from build123d import *

# Parameters (mm, degrees)
CYLINDER016_R          = 3
CYLINDER016_DEPTH      = 20
CYLINDER016_ROLL_ANGLE = 90
CYLINDER015_R          = 3
CYLINDER015_DEPTH      = 20
CYLINDER015_ROLL_ANGLE = 90
BOX016_W               = 40
BOX016_H               = 40
BOX016_DEPTH           = 25
BOX016_ROLL_ANGLE      = 90


with BuildPart() as cylinder016:
    # Cylinder016 → Cylinder016 (new body)
    with BuildSketch(Plane.XY):
        Circle(CYLINDER016_R)
    extrude(amount=CYLINDER016_DEPTH)


with BuildPart() as cylinder016_1:
    # Cylinder016 roll: moved
    add(cylinder016.part.rotate(Axis((0, 0, 0), (1, 0, 0)), CYLINDER016_ROLL_ANGLE))


with BuildPart() as cylinder016_2:
    # Cylinder016 placement: moved
    add(cylinder016_1.part.moved(Location((162, -7, 145))))


with BuildPart() as cylinder015:
    # Cylinder015 → Cylinder015 (new body)
    with BuildSketch(Plane.XY):
        Circle(CYLINDER015_R)
    extrude(amount=CYLINDER015_DEPTH)


with BuildPart() as cylinder015_1:
    # Cylinder015 roll: moved
    add(cylinder015.part.rotate(Axis((0, 0, 0), (1, 0, 0)), CYLINDER015_ROLL_ANGLE))


with BuildPart() as cylinder015_2:
    # Cylinder015 placement: moved
    add(cylinder015_1.part.moved(Location((178, -7, 145))))


with BuildPart() as cut009:
    # Box016 → Box016 (new body)
    with BuildSketch(Plane.XY):
        with Locations((20, 20)):
            Rectangle(BOX016_W, BOX016_H)
    extrude(amount=BOX016_DEPTH)


with BuildPart() as cut009_1:
    # Box016 roll: moved
    add(cut009.part.rotate(Axis((0, 0, 0), (1, 0, 0)), BOX016_ROLL_ANGLE))


with BuildPart() as cut009_2:
    # Box016 placement: moved
    add(cut009_1.part.moved(Location((150, 0, 125))))

    # Cut008: cut Cylinder015
    add(cylinder015_2.part, mode=Mode.SUBTRACT)

    # Cut009: cut Cylinder016
    add(cylinder016_2.part, mode=Mode.SUBTRACT)


with BuildPart() as cut009_3:
    # Cut009 placement: moved
    add(cut009_2.part.moved(Location((0, 20, 0))))


solid = cut009_3.part
Source: CAD feature listing. Evaluate the final solid. Frame: model axes, mm. A direction names the side the tool comes from. Give positions to 0.01 mm unless a question says otherwise; leave off trailing zeros. Order: outer loops, then holes, each group sorted by start corner. A loop starts at its lowest first (then second) coordinate and runs counter-clockwise, first axis right, second up. Notation, with made-up numbers: (-36.75, 35) -> (17.25, 35) arc R22 cw to (17.25, 54) -> close; hole circle Ø7 at (57.25, 67.5). An arc over 180 degrees is marked (long way). Use a Markdown table: item, result.
1) Reachability of faces 5 (the flat face through (150, 8, 145)), 6 (the flat face through (162, 13, 145)) from +Z, -Z, +X, -X, +Y, -Y: full face, straight path, thin tool, end or side. Return the list, or none.
Answer list:
| item | result |
|---|---|
| face 5 | +Z, -Z, -X, +Y, -Y |
| face 6 | -Y |
2) Section query A-A, the plane z = 145. Return the cut outline in (x, y).
Answer list:
| item | result |
|---|---|
| outline | (150, -5) -> (159, -5) -> (159, 13) -> (165, 13) -> (165, -5) -> (175, -5) -> (175, 13) -> (181, 13) -> (181, -5) -> (190, -5) -> (190, 20) -> (150, 20) -> close |
3) Section query B-B, the plane y = -1.5. Return the cut outline in (x, z), then the cut area to 3 significant figures.
Answer list:
| item | result |
|---|---|
| outline | (150, 125) -> (190, 125) -> (190, 165) -> (150, 165) -> close; hole circle Ø6 at (162, 145); hole circle Ø6 at (178, 145) |
| area | 1,540 mm² |
4) Section query D-D, the plane x = 176. Return the cut outline in (y, z), then the cut area to 4 significant figures.
Answer list:
| item | result |
|---|---|
| outline | (-5, 125) -> (20, 125) -> (20, 165) -> (-5, 165) -> (-5, 147.24) -> (13, 147.24) -> (13, 142.76) -> (-5, 142.76) -> close |
| area | 919.5 mm² |
5) Section query C-C, the plane x = 162. Return the cut outline in (y, z), then the cut area to 3 significant figures.
Answer list:
| item | result |
|---|---|
| outline | (-5, 125) -> (20, 125) -> (20, 165) -> (-5, 165) -> (-5, 148) -> (13, 148) -> (13, 142) -> (-5, 142) -> close |
| area | 892 mm² |
6) Contact query for flat-ended pins moving along their axis: P1, Ø3.5, axis at x = 162, z = 145, coming from the -Y side; P2, Ø7, axis at x = 178, z = 145, coming from the -Y side. Output: stop coordinate, or through.
Answer list:
| item | result |
|---|---|
| P1 | y = 13 |
| P2 | y = -5 |
7) Ray query, line 1 along X through (y, z) = (4.75, 145); line 2 along Z through (x, y) = (162, -1.5); line 3 along Z through (x, y) = (160, 7). Return the intervals inside material, ascending. Write a range as [from, to].
Answer list:
| item | result |
|---|---|
| line 1 | [150, 159], [165, 175], [181, 190] |
| line 2 | [125, 142], [148, 165] |
| line 3 | [125, 142.76], [147.24, 165] |
8) Mould query, pull axis Z, two halves, no side actions, for faces 1 (the flat face through (170, 8, 165)), 2 (the flat face through (170, 8, 125)), 3 (the flat face through (170, -5, 145)), 4 (the cylindrical face through (163.61, 4.13, 147.53)). Classes: +Z half, -Z half, draft (parallel to the pull), parting line (faces both ways), or undercut.
Answer list:
| item | result |
|---|---|
| face 1 | +Z half |
| face 2 | -Z half |
| face 3 | draft |
| face 4 | undercut |
